Autodesk Inventor part; units mm, degrees
ref_plane "YZ Plane" through (0, 0, 0) normal (1, 0, 0) x (0, 1, 0)
ref_plane "XZ Plane" through (0, 0, 0) normal (0, 1, 0) x (-1, 0, 0)
ref_plane "XY Plane" through (0, 0, 0) normal (0, 0, 1) x (1, 0, 0)
sketch "草圖1" plane through (0, 0, 0) normal (0, 0, 1) x (1, 0, 0)
  line L0 (0, 0) -> (50, 0)
  line L1 (50, 0) -> (50, 15)
  line L2 (50, 15) -> (0, 15)
  line L3 (0, 15) -> (0, 0)
  circle A0 centre (57.5, 7.5) radius 7.5
  line L4 (50, 15) -> (57.5, 15)
  line L5 (50, 0) -> (57.5, 0)
  circle A1 centre (57.5, 7.5) radius 4
  arc A2 (-63.5, 97) -> (33.5, 0) centre (33.5, 97) ccw
  line L6 (33.5, 0) -> (53.5, 0)
  line L7 (53.5, 7.5) -> (53.5, 0)
  point P0 (0, 5.9684)
  point P1 (33.5, 0)
  dimension "d3" = 8
  dimension "d0" = 50
  dimension "d1" = 15
  dimension "d2" = 15
  dimension "d6" = 20
  dimension "d7" = 97
  dimension "d8" = 137.1787
extrude "擠出1" add sketch "草圖1" along normal blind 3 contours A2 L3 L2 L1 L0 | L1 A0 L7 L5 | L1 L4 A0 | A0 | L7 A0 L5
Here's how the part is built. I have some questions about the finished solid (model axes, mm). Give positions to 0.01 mm unless a question says otherwise; leave off trailing zeros. Loops run counter-clockwise (first coordinate to the right, second up) from the corner with the lowest first, then second, coordinate; pieces in that order, holes last. Notation, with made-up numbers: M 20,-37.75 L 25,-37.75 A20 cw 25,-29.75 Z; hole C 28.25,-14 d8. An arc over 180 degrees is marked long. Put each result on its own line as item: value. Start each with the question number.
(1) I want a section at C-C on y = 13.5. Please give me the cut outline in (x, z).
(2) I want a section at B-B on z = 2.4. Please give me the cut outline in (x, y).
(3) I need wall thicknesses on line 1 along Y through (x, z) = (57.5, 0.9); line 2 along X through (y, z) = (7.5, 0.8); line 3 along X through (y, z) = (8.75, 0.9). Which ranges of each line are inside material? Lowest first, please. Write a range as [from, to].
(4) If we mould it in two halves opening along Y, with no side actions, what happens to faces 1 (the flat face through (45, 0, 1)), 2 (the cylindrical face through (61.315, 6.299, 1.479)), 3 (the flat face through (29, 15, 1))? For each: +Y half, -Y half, draft (parallel to the pull), parting line (faces both ways), or undercut.
(5) I want a section at A-A on y = 7.5. Please give me the cut outline in (x, z), then the cut area to 3 significant figures.
(6) I want a section at D-D on y = 10. Please give me the cut outline in (x, z), then the cut area to 3 significant figures.
Answer block:
1. outline: M 0,0 L 62,0 L 62,3 L 0,3 Z
2. outline: M 0,5.97 A97 ccw 33.5,0 L 57.5,0 A7.5 ccw 57.5,15 L 0,15 Z; hole C 57.5,7.5 d8
3. line 1: [0, 3.5], [11.5, 15]
3. line 2: [0, 53.5], [61.5, 65]
3. line 3: [0, 53.7], [61.3, 64.9]
4. face 1: -Y half
4. face 2: undercut
4. face 3: +Y half
5. outline: M 0,0 L 53.5,0 L 53.5,3 L 0,3 Z; M 61.5,0 L 65,0 L 65,3 L 61.5,3 Z
5. area: 171 mm^2
6. outline: M 0,0 L 54.38,0 L 54.38,3 L 0,3 Z; M 60.62,0 L 64.57,0 L 64.57,3 L 60.62,3 Z
6. area: 175 mm^2
